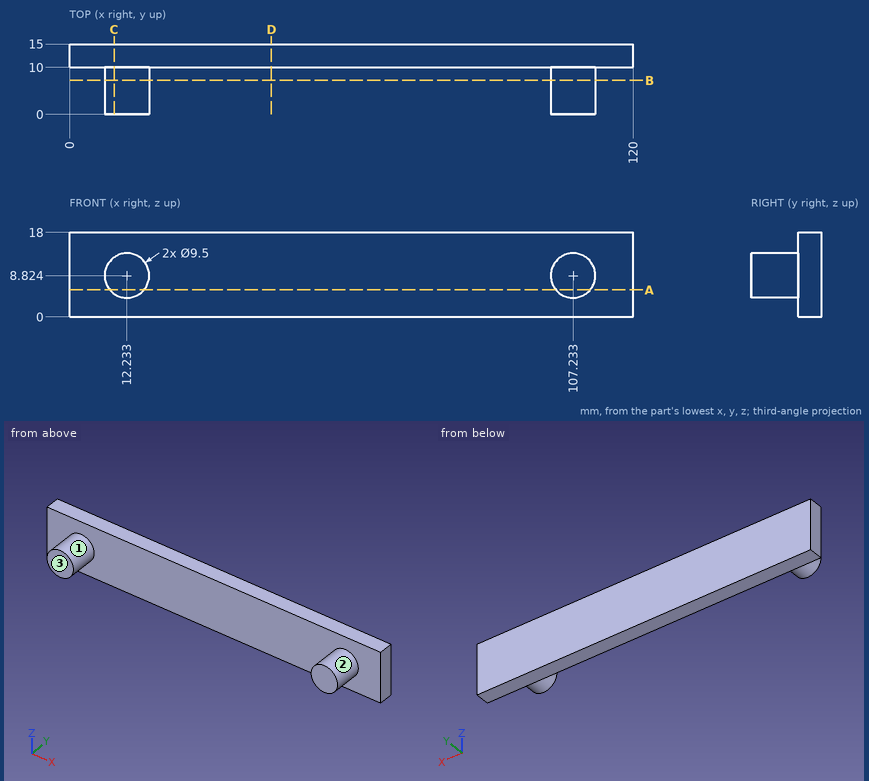
Geometry check sheet. Reference: drawing and pictorial views, mm from the part's lowest x, y, z. Round coordinates to 2 decimals unless told otherwise and drop trailing zeros. Order: outer loops, then holes, each group sorted by start corner. A loop starts at its lowest first (then second) coordinate and runs counter-clockwise, first axis right, second up. Notation, with made-up numbers: (41, 38) - (73, 38) arc R23 cw to (73, 63) - close; hole circle Ø10 at (86.5, 28). An arc over 180 degrees is marked (long way). Use a Markdown table: item, result. Add a question column.
1) Section check C-C (x = 9.5). Record the cut outline in (y, z).
2) Thickness scan on line 1 along Y through (x, z) = (60, 10); line 2 along X through (y, z) = (2.5, 12.75) (1 decimal); line 3 along X through (y, z) = (6.5, 7.75) (1 decimal). Record the ranges inside material, lowest first.
3) Gauge pin test, flat ends, axial feed: P1, Ø5, axis at x = 66, y = 12, coming from the -Z side; P2, Ø4, axis at y = 6.5, z = 4.5, coming from the +X side (1 decimal). Record the tip position at first contact, or that the pin passes through.
4) Section check B-B (y = 7.25). Record the cut outline in (x, z).
5) Section check A-A (z = 5.75). Record the cut outline in (x, y).
6) Mould release check, pull along X, two halves, no side actions. Record for the marked faces 1, 2 and 3: released by +X, released by -X, zero draft, split by the parting line, or undercut.
7) Section check D-D (x = 43). Record the cut outline in (y, z), then the cut area to 3 significant figures.
Established:
| question | item | result |
|---|---|---|
| 1 | outline | (0, 4.94) - (10, 4.94) - (10, 0) - (15, 0) - (15, 18) - (10, 18) - (10, 12.71) - (0, 12.71) - close |
| 2 | line 1 | 10 to 15 |
| 2 | line 2 | 9.6 to 14.9, 104.6 to 109.9 |
| 2 | line 3 | 7.6 to 16.9, 102.6 to 111.9 |
| 3 | P1 | z = 0 |
| 3 | P2 | x = 111.4 |
| 4 | outline | circle Ø9.5 at (12.23, 8.82); circle Ø9.5 at (107.23, 8.82) |
| 5 | outline | (0, 10) - (8.61, 10) - (8.61, 0) - (15.85, 0) - (15.85, 10) - (103.61, 10) - (103.61, 0) - (110.85, 0) - (110.85, 10) - (120, 10) - (120, 15) - (0, 15) - close |
| 6 | face 1 | undercut |
| 6 | face 2 | undercut |
| 6 | face 3 | zero draft |
| 7 | outline | (10, 0) - (15, 0) - (15, 18) - (10, 18) - close |
| 7 | area | 90.0 mm2 |
